Build history of the part. All positions in model axes, mm. Give positions to 0.01 mm unless a question says otherwise; leave off trailing zeros. Write each loop counter-clockwise with the first axis right and the second up, starting at its lowest first coordinate (ties: lowest second). Pieces come first, ordered by that corner, then holes. Notation, with made-up numbers: (-29.75, 20.5) -> (-24.75, 20.5) arc R28 cw to (-24.75, 43.5) -> close; hole circle Ø9 at (36, 67). An arc over 180 degrees is marked (long way). Write item = value, one per line. Start each with the question number.
Q1. Drop flat-ended pins along their axis: P1, Ø1.5, axis at x = -18, y = -12.5, coming from the +Z side; P2, Ø2, axis at x = -39, y = -83.5, coming from the +Z side; P3, Ø2, axis at x = -1.5, y = -82, coming from the -Z side. Give the stop position or say it passes through.
Q2. Mould opens along Z. For faces 1 (the face through (-11.35, -115.11, -51.09)), 2 (the face through (21.361, -59.402, 33.504)), 3 (the face through (23, 0, 39)) say: pulls with the +Z half, pulls with the -Z half, needs draft (parallel to the pull), parting line crosses it, or undercut.
Q3. Saw through at B-B, the plane x = 0. List the corners of the cut face in (y, z).
Q4. Saw through at C-C, the plane y = -103. List the corners of the cut face in (x, z).
Q5. Saw through at A-A, the plane z = 0. List the corners of the cut face in (x, y).
Q6. Wall check: line 1 (Z direction, x = 0, y = -38); line 2 (X direction, y = -83.5, z = 32); line 3 (X direction, y = -14.5, z = 24.5). Give the ranges that are in metal, low to high.
from build123d import *

# Parameters (mm, degrees)
F0_R     = 57.09467
F0_R_2   = 39.73405
F1_DEPTH = 115.348577
F2_SIZE  = 5
F3_R     = 5
F4_R     = 5


with BuildPart() as f1:
    # F0 (on Front) → F1 (new body)
    with BuildSketch(Plane.XZ):
        Circle(F0_R)
        Circle(F0_R_2, mode=Mode.SUBTRACT)
    extrude(amount=F1_DEPTH)

    # F2
    f2_edges = [f1.edges().sort_by_distance(p)[0] for p in [
        (-57.09467, -115.348577, 0),
    ]]
    chamfer(f2_edges, length=F2_SIZE)

    # F3
    f3_edges = [f1.edges().sort_by_distance(p)[0] for p in [
        (-57.09467, 0, 0),
    ]]
    fillet(f3_edges, radius=F3_R)

    # F4
    f4_edges = [f1.edges().sort_by_distance(p)[0] for p in [
        (-39.73405, 0, 0),
    ]]
    fillet(f4_edges, radius=F4_R)


solid = f1.part
Report:
q1.P1 = 54.43
q1.P2 = 42.61
q1.P3 = -57.09
q2.face_1 = parting line crosses it
q2.face_2 = undercut
q2.face_3 = needs draft
q3.outline = (-115.35, -52.09) -> (-110.35, -57.09) -> (-5, -57.09) arc R5 ccw to (0, -52.09) -> (0, -44.73) arc R5 ccw to (-5, -39.73) -> (-115.35, -39.73) -> close; (-115.35, 39.73) -> (-5, 39.73) arc R5 ccw to (0, 44.73) -> (0, 52.09) arc R5 ccw to (-5, 57.09) -> (-110.35, 57.09) -> (-115.35, 52.09) -> close
q4.outline = circle Ø114.19 at (0, 0); hole circle Ø79.47 at (0, 0)
q5.outline = (-57.09, -110.35) -> (-52.09, -115.35) -> (-39.73, -115.35) -> (-39.73, -5) arc R5 ccw to (-44.73, 0) -> (-52.09, 0) arc R5 ccw to (-57.09, -5) -> close; (39.73, -115.35) -> (52.09, -115.35) -> (57.09, -110.35) -> (57.09, -5) arc R5 ccw to (52.09, 0) -> (44.73, 0) arc R5 ccw to (39.73, -5) -> close
q6.line_1 = -57.09 to -39.73, 39.73 to 57.09
q6.line_2 = -47.28 to -23.55, 23.55 to 47.28
q6.line_3 = -51.57 to -31.28, 31.28 to 51.57
